Could you check a few things on this model? Use its own coordinates, in mm. Face numbers are marked on the shaded views. A direction names the side the tool comes from. Give positions to 0.01 mm unless a question says otherwise; leave off trailing zeros. Loops run counter-clockwise (first coordinate to the right, second up) from the corner with the lowest first, then second, coordinate; pieces in that order, holes last. Notation, with made-up numbers: (-39, 89) - (9, 89) arc R33 ccw to (9, 124) - close; hole circle Ø2 at (-20, 3). An arc over 180 degrees is marked (long way). One line per item, written item: value. Start each with the question number.
Q1. For the marked faces 1, 2, 3 and 4, which set-ups out of +Z, -Z, +X, -X, +Y, -Y let a thin tool reach every point of the face, with its end or its side?
Q2. If we mould it in two halves opening along X, with no side actions, what happens to the marked faces 5, 6, 7 and 8? For each: released by +X, released by -X, zero draft, split by the parting line, or undercut.
Q3. I want a section at D-D (x = 74). Please give me the cut outline in (y, z), then the cut area to 3 significant figures.
Q4. I want a section at A-A (z = -6.5). Please give me the cut outline in (x, y).
Q5. If I drill on line 1 (Z direction, x = 120.5, y = 11); line 2 (Z direction, x = -37.5, y = 50.5); line 3 (Y direction, x = 137.5, z = 60), over which ranges is the centre line in solid material (lowest first)? Write a range as from..to.
Q6. I want a section at C-C (y = -46). Please give me the cut outline in (x, z).
Q7. I'm going to push flat-ended pins straight in: P1, Ø15, axis at x = 96.5, y = 1.5, coming from the -Z side; P2, Ø5, axis at x = 20.5, z = 33.5, coming from the +Y side; P3, Ø22.5, axis at x = -10.5, y = 25.5, coming from the +Z side; P4, Ø8, axis at x = 124, y = 31.5, coming from the +Z side. Where does each tip first touch, or does it pass through?
Q8. I want a section at B-B (x = 110). Please give me the cut outline in (y, z), then the cut area to 3 significant figures.
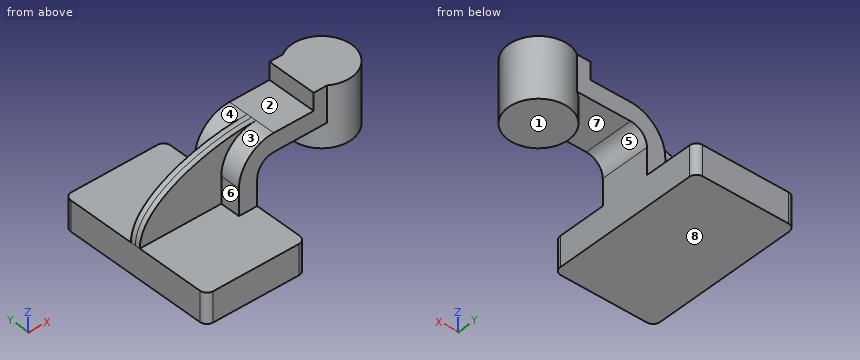
```python
from build123d import *

# Parameters (mm, degrees)
F1_DEPTH = 80
F2_DEPTH = 25
F3_DEPTH = 5
F4_DEPTH = 25
F6_R     = 7


with BuildPart() as f1:
    # F0 (on Front) → F1 (new body, symmetric)
    with BuildSketch(Plane.XZ):
        Polygon((31.686229, 15), (-50, 15), (-50, -15), (50, -15), (50, 15), align=None)
    extrude(amount=F1_DEPTH, both=True)

    # F0 (on Front) → F2 (join, symmetric)
    with BuildSketch(Plane.XZ):
        with BuildLine():
            Line((31.686229, 41.474519), (31.686229, 15))
            Line((31.686229, 15), (50, 15))
            Line((50, 15), (50, 41.474519))
            ThreePointArc((50, 41.474519), (54.850968, 53.185792), (66.562242, 58.03676))
            Line((66.562242, 58.03676), (106.641613, 58.03676))
            Line((106.641613, 58.03676), (106.641613, 76.350532))
            Line((106.641613, 76.350532), (66.562242, 76.350532))
            ThreePointArc((66.562242, 76.350532), (41.901176, 66.135584), (31.686229, 41.474519))
        make_face()
    extrude(amount=F2_DEPTH, both=True)

    # F0 (on Front) → F3 (join, symmetric)
    with BuildSketch(Plane.XZ):
        with BuildLine():
            add(Edge.make_bspline(
                [(-50, 15), (-50, 55.069078), (18.715411, 76.350532), (66.562242, 76.350532)],
                knots=[0, 0, 0, 0, 131.721843, 131.721843, 131.721843, 131.721843], degree=3))
            Line((-50, 15), (31.686229, 15))
            Line((31.686229, 15), (31.686229, 41.474519))
            ThreePointArc((31.686229, 41.474519), (41.901176, 66.135584), (66.562242, 76.350532))
        make_face()
    extrude(amount=F3_DEPTH, both=True)

    # F0 (on Front) → F4 (join, symmetric)
    with BuildSketch(Plane.XZ):
        Polygon((106.641613, 93.709281), (106.641613, 76.350532), (106.641613, 58.03676), (136.641613, 58.03676), (136.641613, 63.709281), (136.641613, 93.709281), align=None)
    extrude(amount=F4_DEPTH, both=True)

    # F0 (on Front) → F5 (revolve)
    with BuildSketch(Plane.XZ):
        Polygon((166.641613, 93.709281), (136.641613, 93.709281), (136.641613, 63.709281), (136.641613, 58.03676), (136.641613, 33.709281), (166.641613, 33.709281), align=None)
    revolve(axis=Axis((136.641613, 0, 78.709281), (0, 0, 1)))

    # F6
    f6_edges = [f1.edges().sort_by_distance(p)[0] for p in [
        (50, -80, 0),
        (-50, -80, 0),
        (50, 80, 0),
        (-50, 80, 0),
    ]]
    fillet(f6_edges, radius=F6_R)


solid = f1.part
```
Worked answers:
1. face 1: -Z, +X, +Y, -Y
1. face 2: +Z, -X, +Y, -Y
1. face 3: +Z, -X, -Y
1. face 4: +Z, -X, +Y
2. face 5: undercut
2. face 6: released by -X
2. face 7: undercut
2. face 8: zero draft
3. outline: (-25, 58.04) - (25, 58.04) - (25, 76.35) - (-25, 76.35) - close
3. area: 916 mm²
4. outline: (-50, -73) arc R7 ccw to (-43, -80) - (43, -80) arc R7 ccw to (50, -73) - (50, 73) arc R7 ccw to (43, 80) - (-43, 80) arc R7 ccw to (-50, 73) - close
5. line 1: z = 33.71..93.71
5. line 2: z = -15..15
5. line 3: y = -29.99..29.99
6. outline: (-50, -15) - (50, -15) - (50, 15) - (-50, 15) - close
7. P1: stops at z = 58.04
7. P2: stops at y = 5
7. P3: stops at z = 15
7. P4: stops at z = 93.71
8. outline: (-25, 58.04) - (-13.79, 58.04) - (-13.79, 33.71) - (13.79, 33.71) - (13.79, 58.04) - (25, 58.04) - (25, 93.71) - (-25, 93.71) - close
8. area: 2,450 mm²
